Drawing for the job (mm, zero at the part's lowest x, y, z). Give positions to 0.01 mm unless a question says otherwise; leave off trailing zeros. Order: outer loops, then holes, each group sorted by start corner. A loop starts at its lowest first (then second) coordinate and runs counter-clockwise, first axis right, second up. Notation, with made-up numbers: (-10, 67) -> (-5, 67) arc R29 cw to (-5, 91) -> close; hole circle Ø9 at (80.25, 78.25). An arc over 180 degrees is marked (long way). Use one line per item in the form item = value. Start each with the question number.
1) Cut at D-D, the plane y = 3.05. State how many separate pieces and enclosed holes the cut face has, and give its area (3 significant figures).
2) Probe line 1 (Z direction, x = 39, y = 0.85) (1 decimal); line 2 (Z direction, x = 38, y = 1.2); line 3 (X direction, y = 0.45, z = 47) (1 decimal). List the from-to ranges inside material, lowest first.
3) Cut at C-C, the plane x = 39.5. Give the cut face in (y, z), and give its area (3 significant figures).
4) Cut at B-B, the plane z = 18. Give the cut face in (x, y).
5) Cut at A-A, the plane x = 20.5. Give the cut face in (y, z).
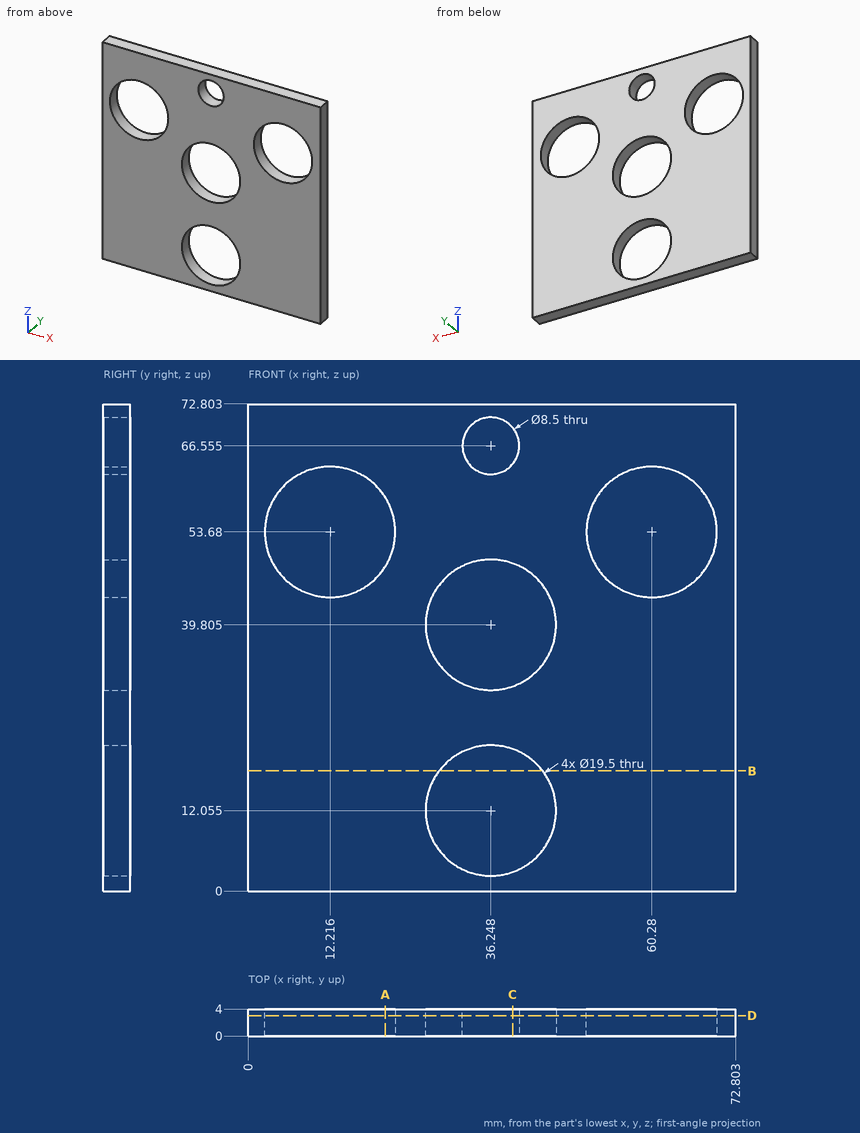
Result:
q1.separate_pieces = 1
q1.enclosed_holes = 5
q1.area = 4,050 mm²
q2.line_1 = 0 to 2.7, 21.4 to 30.5, 49.2 to 63.3, 69.8 to 72.8
q2.line_2 = 0 to 2.46, 21.65 to 30.21, 49.4 to 62.68, 70.43 to 72.8
q2.line_3 = 0 to 5.1, 19.3 to 29.7, 42.8 to 53.2, 67.4 to 72.8
q3.outline = (0, 0) -> (4, 0) -> (4, 2.86) -> (0, 2.86) -> close; (0, 21.25) -> (4, 21.25) -> (4, 30.61) -> (0, 30.61) -> close; (0, 49) -> (4, 49) -> (4, 63.82) -> (0, 63.82) -> close; (0, 69.29) -> (4, 69.29) -> (4, 72.8) -> (0, 72.8) -> close
q3.area = 122 mm²
q4.outline = (0, 0) -> (28.52, 0) -> (28.52, 4) -> (0, 4) -> close; (43.98, 0) -> (72.8, 0) -> (72.8, 4) -> (43.98, 4) -> close
q5.outline = (0, 0) -> (4, 0) -> (4, 48.54) -> (0, 48.54) -> close; (0, 58.82) -> (4, 58.82) -> (4, 72.8) -> (0, 72.8) -> close
